from build123d import *

# Parameters (mm, degrees)
BOSS_EXTRUDE1_DEPTH = 28.5
SKETCH2_R           = 23
BOSS_EXTRUDE2_DEPTH = 78
SKETCH3_R           = 9.125
BOSS_EXTRUDE3_DEPTH = 6
SKETCH4_R           = 3.5
BOSS_EXTRUDE4_DEPTH = 25
CUT_EXTRUDE1_START  = -18
CUT_EXTRUDE1_DEPTH  = 18
SKETCH6_R           = 2.4
CUT_EXTRUDE2_DEPTH  = 10
SKETCH7_R           = 12.5
SKETCH7_R_2         = 9.125
BOSS_EXTRUDE5_DEPTH = 3


with BuildPart() as part:
    # Sketch1 → Boss-Extrude1 (new body)
    with BuildSketch(Plane.XY):
        with BuildLine():
            Line((5, 0), (55, 0))
            ThreePointArc((55, 0), (58.535533906, 1.464466094), (60, 5))
            Line((60, 5), (60, 55))
            ThreePointArc((60, 55), (58.535533906, 58.535533906), (55, 60))
            Line((55, 60), (5, 60))
            ThreePointArc((5, 60), (1.464466094, 58.535533906), (0, 55))
            Line((0, 55), (0, 5))
            ThreePointArc((0, 5), (1.464466094, 1.464466094), (5, 0))
        make_face()
    extrude(amount=BOSS_EXTRUDE1_DEPTH)

    # Sketch2 → Boss-Extrude2 (add)
    with BuildSketch(Plane.XY.offset(28.5)):
        with Locations((30, 30)):
            Circle(SKETCH2_R)
    extrude(amount=BOSS_EXTRUDE2_DEPTH)

    # Sketch3 → Boss-Extrude3 (add)
    with BuildSketch(Plane(origin=(0, 0, 0), x_dir=(-1, 0, 0), z_dir=(0, 0, -1))):
        with Locations((-30, 40)):
            Circle(SKETCH3_R)
    extrude(amount=BOSS_EXTRUDE3_DEPTH)

    # Sketch4 → Boss-Extrude4 (add)
    with BuildSketch(Plane(origin=(0, 0, -6), x_dir=(-1, 0, 0), z_dir=(0, 0, -1))):
        with Locations((-30, 42.25)):
            Circle(SKETCH4_R)
    extrude(amount=BOSS_EXTRUDE4_DEPTH)

    # Sketch5 → Cut-Extrude1 (cut)
    with BuildSketch(Plane(origin=(0, 0, -31), x_dir=(-1, 0, 0), z_dir=(0, 0, -1)).offset(CUT_EXTRUDE1_START)):
        with BuildLine():
            Line((-32.5, 39.800510257), (-27.5, 39.800510257))
            ThreePointArc((-27.5, 39.800510257), (-30, 38.75), (-32.5, 39.800510257))
        make_face()
    extrude(amount=CUT_EXTRUDE1_DEPTH, mode=Mode.SUBTRACT)

    # Sketch6 → Cut-Extrude2 (cut)
    with BuildSketch(Plane(origin=(0, 0, 0), x_dir=(-1, 0, 0), z_dir=(0, 0, -1))):
        with Locations((-54.75, 54.75)):
            Circle(SKETCH6_R)
        with Locations((-5.25, 54.75)):
            Circle(SKETCH6_R)
        with Locations((-5.25, 5.25)):
            Circle(SKETCH6_R)
        with Locations((-54.75, 5.25)):
            Circle(SKETCH6_R)
    extrude(amount=-CUT_EXTRUDE2_DEPTH, mode=Mode.SUBTRACT)

    # Sketch7 → Boss-Extrude5 (add)
    with BuildSketch(Plane(origin=(0, 0, 0), x_dir=(-1, 0, 0), z_dir=(0, 0, -1))):
        with Locations((-30, 40)):
            Circle(SKETCH7_R)
        with Locations((-30, 40)):
            Circle(SKETCH7_R_2, mode=Mode.SUBTRACT)
    extrude(amount=BOSS_EXTRUDE5_DEPTH)


solid = part.part
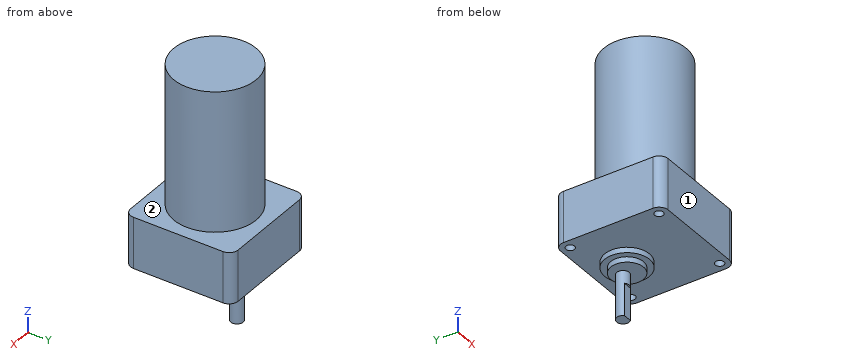
Could you check a few things on this model? Use its own coordinates, in mm. Face numbers are marked on the shaded views. A direction names the side the tool comes from. Coordinates: 2 decimals unless noted, no trailing zeros. Order: outer loops, then holes, each group sorted by start corner. A loop starts at its lowest first (then second) coordinate and runs counter-clockwise, first axis right, second up.
Q1. Suppose I cut it at B-B on x = 47.5. Please give me the cut outline in (y, z).
Q2. Suppose I cut it at D-D on y = 42.25. Please give me the cut outline in (x, z).
Q3. Suppose I cut it at C-C on z = 94.5. Please give me the cut outline in (x, y), and give its area (3 significant figures).
Q4. Will these pins go through, and if not, where does the flat tip stop? pin 1 (3 mm diameter, centred on x = 20, y = 27.5, fed in from -Z); pin 2 (3 mm diameter, centred on x = 25, y = 27, fed in from -Z); pin 3 (1 mm diameter, centred on x = 35, y = 32, fed in from -Z).
Q5. Suppose I cut it at A-A on y = 24.5. Please give me the cut outline in (x, z).
Q6. Which directions (+Z, -Z, +X, -X, +Y, -Y) give clear straight access to the entire face, cutting with the end or side of a thin tool? Please do the marked faces 1 and 2.
Q7. Please list where these lines run through material, in increasing order: L1, parallel to Y at x = 5.25, z = 2; L2, parallel to X at y = 5, z = 4; L3, parallel to Y at x = 54, z = 5.
Answer:
1. outline: (0, 0) - (60, 0) - (60, 28.5) - (44.92, 28.5) - (44.92, 106.5) - (15.08, 106.5) - (15.08, 28.5) - (0, 28.5) - close
2. outline: (0, 0) - (17.7, 0) - (17.7, -3) - (21.16, -3) - (21.16, -6) - (26.5, -6) - (26.5, -31) - (33.5, -31) - (33.5, -6) - (38.84, -6) - (38.84, -3) - (42.3, -3) - (42.3, 0) - (60, 0) - (60, 28.5) - (49.47, 28.5) - (49.47, 106.5) - (10.53, 106.5) - (10.53, 28.5) - (0, 28.5) - close
3. outline: circle Ø46 at (30, 30)
3. area: 1,660 mm2
4. pin 1: stops at z = 0
4. pin 2: stops at z = -3
4. pin 3: stops at z = -6
5. outline: (0, 0) - (60, 0) - (60, 28.5) - (52.33, 28.5) - (52.33, 106.5) - (7.67, 106.5) - (7.67, 28.5) - (0, 28.5) - close
6. face 1: +Z, -Z, +X, -X, -Y
6. face 2: +Z
7. L1: y = 0 to 2.85, 7.65 to 52.35, 57.15 to 60
7. L2: x = 0 to 2.86, 7.64 to 52.36, 57.14 to 60
7. L3: y = 0 to 2.97, 7.53 to 52.47, 57.03 to 60
